from build123d import *

# Parameters (mm, degrees)
BOSS_EXTRUDE1_DEPTH                           = 9.5
CBORE_FOR_M12_HEX_HEAD_CAP_SCREW2_D           = 6.75
CBORE_FOR_M12_HEX_HEAD_CAP_SCREW2_CBORE_D     = 25
CBORE_FOR_M12_HEX_HEAD_CAP_SCREW2_CBORE_DEPTH = 5
SCALE1_SCALE                                  = 0.51948


with BuildPart() as part:
    # Sketch1 → Boss-Extrude1 (new, symmetric)
    with BuildSketch(Plane(origin=(0, 0, 0), x_dir=(0, 0, -1), z_dir=(1, 0, 0))):
        with BuildLine():
            ThreePointArc((-12.7, 0), (0, 12.7), (12.7, 0))
            Line((12.7, 0), (25.4, 0))
            Line((25.4, 0), (25.4, 19))
            Line((25.4, 19), (-25.4, 19))
            Line((-25.4, 19), (-25.4, 0))
            Line((-25.4, 0), (-12.7, 0))
        make_face()
    extrude(amount=BOSS_EXTRUDE1_DEPTH, both=True)

    # CBORE for M12 Hex Head Cap Screw2 (through all)
    with Locations(Plane(origin=(0, 19, 0), x_dir=(1, 0, 0), z_dir=(0, 1, 0))):
        with Locations((0, 19.05), (0, -19.05)):
            CounterBoreHole(CBORE_FOR_M12_HEX_HEAD_CAP_SCREW2_D / 2, CBORE_FOR_M12_HEX_HEAD_CAP_SCREW2_CBORE_D / 2, CBORE_FOR_M12_HEX_HEAD_CAP_SCREW2_CBORE_DEPTH)


with BuildPart() as part_1:
    # Scale1: scaled about (0, 9.391105983, 0)
    add(part.part.scale(SCALE1_SCALE).moved(Location((0, 4.512614247, 0))))


solid = part_1.part
The listing builds one solid part. Answer for the finished solid, in the listing's coordinates (mm). A direction names the side the tool comes from. Coordinates: 2 decimals unless noted, no trailing zeros. Write each loop counter-clockwise with the first axis right and the second up, starting at its lowest first coordinate (ties: lowest second). Pieces come first, ordered by that corner, then holes. Notation, with made-up numbers: M 27,85 L 62,85 A23 ccw 62,110 Z; hole C 86.5,33 d8. An arc over 180 degrees is marked long. Put each result on its own line as item: value. Start each with the question number.
1. For a pull along Z with two mould halves and no side action, classify faces 1 (the flat face through (0, 8, -13.195)), 2 (the cylindrical face through (0.228, 8.098, -11.634)), 3 (the flat face through (1, 11.785, 8)) as pulls with the +Z half, pulls with the -Z half, needs draft (parallel to the pull), parting line crosses it, or undercut.
2. A cutting plane is placed at D-D on y = 6.5. Write down the section's boundary in (x, z).
3. A cutting plane is placed at B-B on y = 9.5. Write down the section's boundary in (x, z).
4. Which of the six approach directions +Z, -Z, +X, -X, +Y, -Y give full straight-line access (tool end or side, diameter ignored) to faces 4 (the cylindrical face through (0.23, 8.1, 8.16)), 5 (the cylindrical face through (0.078, 13.102, 3.403)), 6 (the cylindrical face through (-0.078, 13.102, -3.403))?
5. Consider line 1 (Z direction, x = 0, y = 8.25); line 2 (Y direction, x = 3, z = -10.5); line 3 (Z direction, x = -4.25, y = 8.25). Determine where each line is inside the solid, lowest interval first. Write a range as from..to.
6. A flat-ended cylindrical pin translates along its axis: P1, Ø1.5, axis at x = -2, z = 9.5, coming from the +Y side. Find the tip coordinate at first contact, or state that the pin passes through.
7. A cutting plane is placed at C-C on z = 9.5. Write down the section's boundary in (x, y), then the cut area to 3 significant figures.
8. A cutting plane is placed at A-A on x = 0. Write down the section's boundary in (y, z).
Resolved:
1. face 1: pulls with the -Z half
1. face 2: undercut
1. face 3: needs draft
2. outline: M -4.94,-13.19 L 4.94,-13.19 L 4.94,-6.29 L -4.94,-6.29 Z; M -4.94,6.29 L 4.94,6.29 L 4.94,13.19 L -4.94,13.19 Z; hole C 0,-9.9 d3.51; hole C 0,9.9 d3.51
3. outline: M -4.94,-13.19 L 4.94,-13.19 L 4.94,-4.32 L -4.94,-4.32 Z; M -4.94,4.32 L 4.94,4.32 L 4.94,13.19 L -4.94,13.19 Z; hole C 0,-9.9 d3.51; hole C 0,9.9 d3.51
4. face 4: +Y, -Y
4. face 5: +Z, +Y
4. face 6: -Z, +Y
5. line 1: z = -13.19..-11.65, -8.14..-5.44, 5.44..8.14, 11.65..13.19
5. line 2: y = 4.51..11.79
5. line 3: z = -13.19..-5.44, 5.44..13.19
6. P1: stops at y = 11.79
7. outline: M -4.94,4.51 L -1.71,4.51 L -1.71,11.79 L -4.94,11.79 Z; M 1.71,4.51 L 4.94,4.51 L 4.94,11.79 L 1.71,11.79 Z
7. area: 46.9 mm2
8. outline: M 4.51,-13.19 L 11.79,-13.19 L 11.79,-11.65 L 4.51,-11.65 Z; M 4.51,-8.14 L 11.79,-8.14 L 11.79,-3.4 L 14.38,-3.4 L 14.38,3.4 L 11.79,3.4 L 11.79,8.14 L 4.51,8.14 L 4.51,6.6 A6.6 cw 4.51,-6.6 Z; M 4.51,11.65 L 11.79,11.65 L 11.79,13.19 L 4.51,13.19 Z
